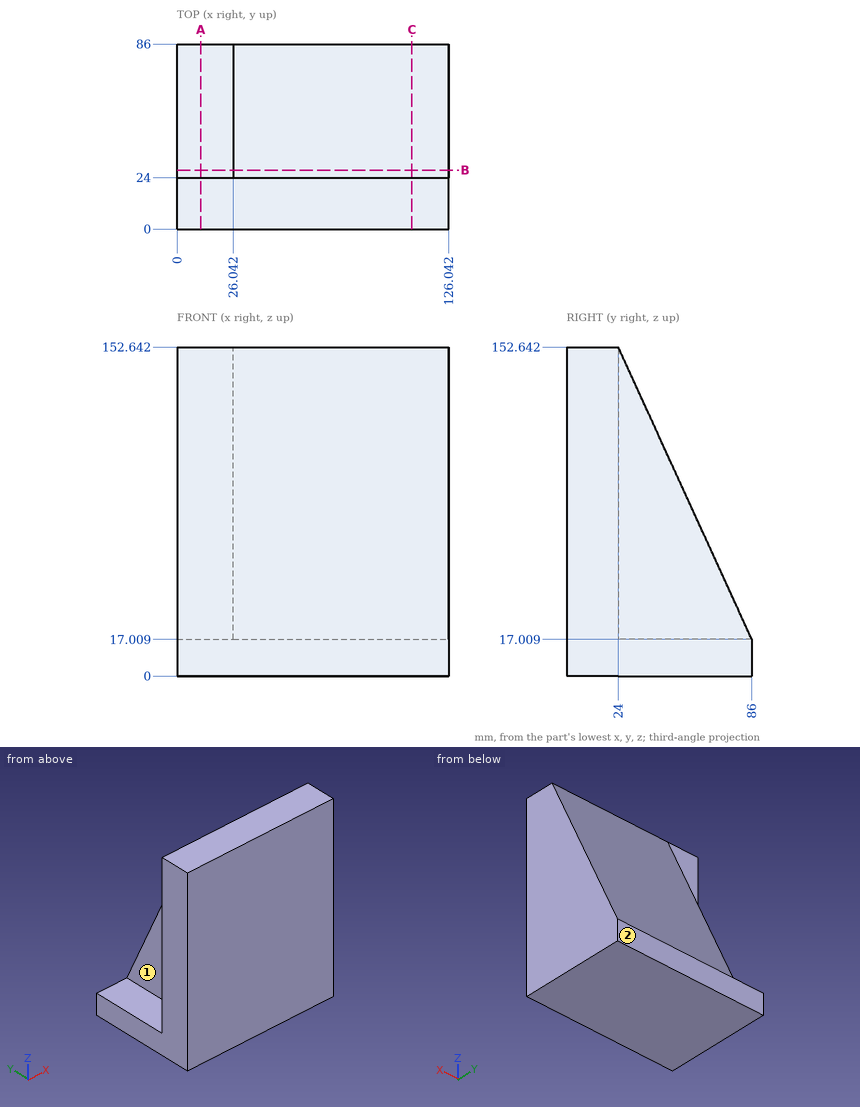
Could you check a few things on this drawing? It's one solid part, dimensions in mm from its lowest x, y, z. A direction names the side the tool comes from. Give positions to 0.01 mm unless a question says otherwise; leave off trailing zeros. Order: outer loops, then holes, each group sorted by start corner. A loop starts at its lowest first (then second) coordinate and runs counter-clockwise, first axis right, second up. Notation, with made-up numbers: (-19.5, 19.25) - (35.5, 19.25) arc R23 cw to (35.5, 46.25) - close; hole circle Ø3 at (-28.75, -26). An arc over 180 degrees is marked (long way). Answer as a JSON object with one key per item and string values. Group by question number.
Item 1: If we section it at B-B on y = 27.5: Please give me the cut outline in (x, z) (1 decimal).
Item 2: For P1, Ø4, axis at x = 73.5, z = 94, coming from the +Y side; P2, Ø3, axis at y = 65.5, z = 49, coming from the -X side; P3, Ø21, axis at x = 15, y = 46.5, coming from the +Z side, each with a flat end and sliding along its axis, tell me the tip position at first contact or that it passes through.
Item 3: Which directions (+Z, -Z, +X, -X, +Y, -Y) give clear straight access to the entire face, cutting with the end or side of a thin tool? Please do the marked faces 1 and 2.
Item 4: If we section it at A-A on x = 11: Please give me the cut outline in (y, z), and give its area (3 significant figures).
Item 5: If we section it at C-C on x = 109: Please give me the cut outline in (y, z).
Item 6: Please list where these lines run through material, in increasing order: probe 1 along Z at (x, y) = (9, 76.5); probe 2 along X at (y, z) = (40.5, 102); probe 3 along Y at (x, z) = (13, 58.5).
Result set:
{
 "1": {"outline": "(0, 0) - (126, 0) - (126, 145) - (26, 145) - (26, 17) - (0, 17) - close"},
 "2": {"P1": "y = 51.72", "P2": "x = 26.04", "P3": "z = 17.01"},
 "3": {"face 1": "+Z, -X, +Y", "face 2": "+Z, -Z, +X, -X, +Y"},
 "4": {"outline": "(0, 0) - (86, 0) - (86, 17.01) - (24, 17.01) - (24, 152.64) - (0, 152.64) - close", "area": "4,720 mm²"},
 "5": {"outline": "(0, 0) - (86, 0) - (86, 17.01) - (24, 152.64) - (0, 152.64) - close"},
 "6": {"probe 1": "0 to 17.01", "probe 2": "26.04 to 126.04", "probe 3": "0 to 24"}
}
